```python
from build123d import *

# Parameters (mm, degrees)
SKETCH_3_R          = 1.5
EXTRUDE_1_DEPTH     = 6
CUT_EXTRUDE_1_DEPTH = 0.5


with BuildPart() as part:
    # 放样1: read off the stored shape, not the designer's step
    # 放样1: loft between two sections, ruled curve by curve
    loft_1_from = [
        Edge.make_bspline([(-2.696565737, 0, 1.314736942), (-0.067091854, 0, 6.707868416), (5.32603962, 0, 4.078394533), (2.696565737, 0, -1.314736942), (0.067091854, 0, -6.707868416), (-5.32603962, 0, -4.078394533), (-2.696565737, 0, 1.314736942)], [0, 0, 0, 0, 0.5, 0.5, 0.5, 1, 1, 1, 1], 3, [1, 0.333333333, 0.333333333, 1, 0.333333333, 0.333333333, 1]),
    ]
    loft_1_to = [
        Edge.make_bspline([(-1.463875143, 2.5, 0.327214862), (-0.809445419, 2.5, 3.254965148), (2.118304867, 2.5, 2.600535424), (1.463875143, 2.5, -0.327214862), (0.809445419, 2.5, -3.254965148), (-2.118304867, 2.5, -2.600535424), (-1.463875143, 2.5, 0.327214862)], [0, 0, 0, 0, 0.5, 0.5, 0.5, 1, 1, 1, 1], 3, [1, 0.333333333, 0.333333333, 1, 0.333333333, 0.333333333, 1]),
    ]
    loft_1 = Solid(Shell([*[Face.make_surface_from_curves(loft_1_from[k], loft_1_to[k]) for k in range(1)], Face(Wire(loft_1_from)), Face(Wire(loft_1_to))]))
    add(loft_1)

    # 草图3 → 凸台-拉伸1 (add)
    with BuildSketch(Plane(origin=(0, 2.5, 0), x_dir=(1, 0, 0), z_dir=(0, 1, 0))):
        with Locations(Location((0, 0, 0), (0, 0, 192.6))):
            Circle(SKETCH_3_R)
    extrude(amount=EXTRUDE_1_DEPTH)

    # 草图4 → 切除-拉伸1 (cut)
    with BuildSketch(Plane.XZ):
        Polygon((0.577350269, 1), (-0.577350269, 1), (-1.154700538, 0), (-0.577350269, -1), (0.577350269, -1), (1.154700538, 0), align=None)
    extrude(amount=-CUT_EXTRUDE_1_DEPTH, mode=Mode.SUBTRACT)


solid = part.part
```
Can you work these out from the model? Positions are in its coordinate system, mm. Round coordinates to 2 decimals unless told otherwise and drop trailing zeros. Loops run counter-clockwise (first coordinate to the right, second up) from the corner with the lowest first, then second, coordinate; pieces in that order, holes last. Notation, with made-up numbers: M -7.5,-12 L 5.5,-12 A37 ccw 5.5,25 Z; hole C 49,27.5 d11. An arc over 180 degrees is marked long. Answer as a JSON object with one key per item and string values. Group by question number.
Q1. Imagine slicing it at A-A, the plane y = 7.5. Please give me the cut outline in (x, z).
Q2. Will these pins go through, and if not, where does the flat tip stop? pin 1 (1 mm diameter, centred on x = 1.5, z = -2.5, fed in from +Y); pin 2 (1.6 mm diameter, centred on x = 0, z = -0.5, fed in from -Y); pin 3 (1.5 mm diameter, centred on y = 1.5, z = 0.5, fed in from +X); pin 4 (3 mm diameter, centred on x = 1.5, y = 4, fed in from +Z).
Q3. Please list where these lines run through material, in increasing order: L1, parallel to X at y = 5.25, z = 0; L2, parallel to Y at x = -0.25, z = -0.5; L3, parallel to X at y = 5, z = 0.75.
Q4. We'd pull the mould along X, two halves only. Please class faces 1 (the flat face through (0, 0.5, 0)), 2 (the cylindrical face through (-1.478, 5.458, -0.258)), 3 (the flat face through (1.2, 0, 0.5)): +X half, -X half, draft (parallel to the pull), parting line (faces both ways), or undercut.
Findings:
{
 "1": {"outline": "C 0,0 d3"},
 "2": {"pin 1": "stops at y = 0.95", "pin 2": "stops at y = 0", "pin 3": "stops at x = 2.51", "pin 4": "stops at z = 1.5"},
 "3": {"L1": "x = -1.5 to 1.5", "L2": "y = 0.5 to 8.5", "L3": "x = -1.3 to 1.3"},
 "4": {"face 1": "undercut", "face 2": "parting line", "face 3": "draft"}
}
